```python
from build123d import *

# Parameters (mm, degrees)
F0_W      = 660
F0_H      = 610
F1_DEPTH  = 120
F2_R      = 80
F4_DEPTH  = 70
F6_DEPTH  = 70
F7_DEPTH  = 70
F8_R      = 62.5
F9_DEPTH  = 10
F10_R     = 40
F11_DEPTH = 180.001
F12_R     = 35
F13_DEPTH = 190.001


with BuildPart() as f1:
    # F0 (on Right) → F1 (new body)
    with BuildSketch(Plane.YZ):
        Rectangle(F0_W, F0_H)
    extrude(amount=F1_DEPTH)

    # F2
    f2_edges = [f1.edges().sort_by_distance(p)[0] for p in [
        (60, 330, 305),
        (60, -330, 305),
        (60, 330, -305),
        (60, -330, -305),
    ]]
    fillet(f2_edges, radius=F2_R)

    # F3 (on face) → F4 (join)
    with BuildSketch(Plane.YZ.offset(120)):
        with BuildLine():
            ThreePointArc((250, 305), (306.5685424949, 281.5685424949), (330, 225))
            Line((330, 225), (330, 305))
            Line((330, 305), (250, 305))
        make_face()
        with BuildLine():
            Line((-330, 305), (-330, 225))
            ThreePointArc((-330, 225), (-306.5685424949, 281.5685424949), (-250, 305))
            Line((-250, 305), (-330, 305))
        make_face()
        with BuildLine():
            Line((-250, -305), (250, -305))
            ThreePointArc((250, -305), (306.5685424949, -281.5685424949), (330, -225))
            Line((330, -225), (330, 225))
            ThreePointArc((330, 225), (306.5685424949, 281.5685424949), (250, 305))
            Line((250, 305), (-250, 305))
            ThreePointArc((-250, 305), (-306.5685424949, 281.5685424949), (-330, 225))
            Line((-330, 225), (-330, -225))
            ThreePointArc((-330, -225), (-306.5685424949, -281.5685424949), (-250, -305))
        make_face()
        with BuildLine():
            Line((250, -305), (330, -305))
            Line((330, -305), (330, -225))
            ThreePointArc((330, -225), (306.5685424949, -281.5685424949), (250, -305))
        make_face()
        with BuildLine():
            Line((-330, -305), (-250, -305))
            ThreePointArc((-250, -305), (-306.5685424949, -281.5685424949), (-330, -225))
            Line((-330, -225), (-330, -305))
        make_face()
    extrude(amount=F4_DEPTH)

    # F5 (on face) → F6 (cut)
    with BuildSketch(Plane.YZ.offset(190)):
        with BuildLine():
            ThreePointArc((-270, 190), (-234.6446609407, 204.6446609407), (-220, 240))
            Line((-220, 240), (-220, 305))
            Line((-220, 305), (-330, 305))
            Line((-330, 305), (-330, 190))
            Line((-330, 190), (-270, 190))
        make_face()
    extrude(amount=-F6_DEPTH, mode=Mode.SUBTRACT)

    # F5 (on face) → F7 (cut)
    with BuildSketch(Plane.YZ.offset(190)):
        with BuildLine():
            Line((330, 305), (220, 305))
            Line((220, 305), (220, 240))
            ThreePointArc((220, 240), (234.6446609407, 204.6446609407), (270, 190))
            Line((270, 190), (330, 190))
            Line((330, 190), (330, 305))
        make_face()
        with BuildLine():
            Line((220, -240), (220, -305))
            Line((220, -305), (330, -305))
            Line((330, -305), (330, -190))
            Line((330, -190), (270, -190))
            ThreePointArc((270, -190), (234.6446609407, -204.6446609407), (220, -240))
        make_face()
        with BuildLine():
            Line((-270, -190), (-330, -190))
            Line((-330, -190), (-330, -305))
            Line((-330, -305), (-220, -305))
            Line((-220, -305), (-220, -240))
            ThreePointArc((-220, -240), (-234.6446609407, -204.6446609407), (-270, -190))
        make_face()
    extrude(amount=-F7_DEPTH, mode=Mode.SUBTRACT)

    # F8 (on face) → F9 (cut)
    with BuildSketch(Plane.YZ.offset(190)):
        Circle(F8_R)
    extrude(amount=-F9_DEPTH, mode=Mode.SUBTRACT)

    # F10 (on face) → F11 (cut, through all)
    with BuildSketch(Plane.YZ.offset(180)):
        Circle(F10_R)
    extrude(amount=-F11_DEPTH, mode=Mode.SUBTRACT)

    # F12 (on face) → F13 (cut, through all)
    with BuildSketch(Plane(origin=(0, 0, 0), x_dir=(0, -1, 0), z_dir=(-1, 0, 0))):
        with Locations((-265, 240)):
            Circle(F12_R)
        with Locations((265, 240)):
            Circle(F12_R)
        with Locations((265, -240)):
            Circle(F12_R)
        with Locations((-265, -240)):
            Circle(F12_R)
    extrude(amount=-F13_DEPTH, mode=Mode.SUBTRACT)


solid = f1.part
```
Geometry: final body of the model. Coordinates: model frame, mm. A direction names the side the tool comes from. Round coordinates to 2 decimals unless told otherwise and drop trailing zeros. Write each loop counter-clockwise with the first axis right and the second up, starting at its lowest first coordinate (ties: lowest second). Pieces come first, ordered by that corner, then holes. Notation, with made-up numbers: (-9, 79.5) -> (-4, 79.5) arc R27 cw to (-4, 117.5) -> close; hole circle Ø4 at (17.25, 67). An arc over 180 degrees is marked (long way). Use CSV: the item, a comma, the result in double quotes. Start each with the question number.
Q1. Line query: L1, parallel to Z at x = 121, y = 0; L2, parallel to Z at x = 185, y = 0; L3, parallel to Z at x = 58, y = -265. Output: solid intervals per line, ascending.
Q2. Section A-A (z = 0). Return loops of the section in (x, y), plus the area to 3 significant figures.
Q3. Reachability of faces 4 (the face through (155.49, 235.036, -204.258)), 5 (the face through (180, -1, -41)), 6 (the face through (155, -220, 272)), 7 (the face through (120, -300, -247)), 8 (the face through (155, 300, 190)) from +Z, -Z, +X, -X, +Y, -Y: full face, straight path, thin tool, end or side. Return the list, or none.
Q4. Pull-direction query (Z, two-part tool) for faces 1 (the face through (94, -4, -305)), 2 (the face through (120, 274, 274)), 3 (the face through (59.16, 246.18, -210.49)); classes: pulls with the +Z half, pulls with the -Z half, needs draft (parallel to the pull), parting line crosses it, or undercut.
Q5. First-contact query: pin 1 Ø18 at (x, y) = (156.5, -299) entering from +Z. Flat tip, straight axial feed; report the tip coordinate or a pass-through.
Q6. Section B-B (y = -241). Return loops of the section in (x, z).
Q7. Section D-D (y = 2.5). Return loops of the section in (x, z), plus the area to 3 significant figures.
Q8. Section C-C (x = 19). Return loops of the section in (y, z).
Result sheet:
1,L1,"-305 to -40, 40 to 305"
1,L2,"-305 to -62.5, 62.5 to 305"
1,L3,"-303.58 to -275, -205 to 205, 275 to 303.58"
2,outline,"(0, -330) -> (190, -330) -> (190, -62.5) -> (180, -62.5) -> (180, -40) -> (0, -40) -> close; (0, 40) -> (180, 40) -> (180, 62.5) -> (190, 62.5) -> (190, 330) -> (0, 330) -> close"
2,area,"110,000 mm²"
3,face 4,"-Z, +X, +Y"
3,face 5,"+X"
3,face 6,"+Z, +X, -Y"
3,face 7,"-Z, +X, -Y"
3,face 8,"+Z, +X, +Y"
4,face 1,"pulls with the -Z half"
4,face 2,"needs draft"
4,face 3,"undercut"
5,pin 1,"z = 190"
6,outline,"(0, -305) -> (120, -305) -> (120, -265.48) -> (0, -265.48) -> close; (0, -214.52) -> (120, -214.52) -> (120, -199.27) -> (190, -199.27) -> (190, 199.27) -> (120, 199.27) -> (120, 214.52) -> (0, 214.52) -> close; (0, 265.48) -> (120, 265.48) -> (120, 305) -> (0, 305) -> close"
7,outline,"(0, -305) -> (190, -305) -> (190, -62.45) -> (180, -62.45) -> (180, -39.92) -> (0, -39.92) -> close; (0, 39.92) -> (180, 39.92) -> (180, 62.45) -> (190, 62.45) -> (190, 305) -> (0, 305) -> close"
7,area,"100,000 mm²"
8,outline,"(-330, -225) arc R80 ccw to (-250, -305) -> (250, -305) arc R80 ccw to (330, -225) -> (330, 225) arc R80 ccw to (250, 305) -> (-250, 305) arc R80 ccw to (-330, 225) -> close; hole circle Ø70 at (-265, -240); hole circle Ø70 at (-265, 240); hole circle Ø80 at (0, 0); hole circle Ø70 at (265, -240); hole circle Ø70 at (265, 240)"
